Design review of the part shown in the three views and the two pictorial views. Dimensions are in mm from the part's minimum x, y and z. A direction names the side the tool comes from. Give positions to 0.01 mm unless a question says otherwise; leave off trailing zeros. Loops run counter-clockwise (first coordinate to the right, second up) from the corner with the lowest first, then second, coordinate; pieces in that order, holes last. Notation, with made-up numbers: (80.5, -12.75) -> (102.5, -12.75) arc R27 ccw to (102.5, 24.25) -> close; hole circle Ø6 at (-9, -22). An arc over 180 degrees is marked (long way). One line per question, with ' | ' between items. Start each with the question number.
(1) Draft analysis for pull direction Y (two halves, no side actions). For the marked faces 1, 2, 3 and 4, state which applies: +Y half, -Y half, draft (parallel to the pull), parting line (faces both ways), or undercut.
(2) Insertion check: P1, Ø2, axis at y = 11.5, z = 12.5, coming from the -X side; P2, Ø3, axis at x = 59.92, y = 6.35, coming from the +Z side; P3, Ø2, axis at x = 60.5, y = 8, coming from the +Z side; P4, Ø3, axis at y = 8, z = 12.5, coming from the -X side (1 decimal). Each pin has a flat end and moves straight along its axis. Give the tip position at first contact, or say it passes through.
(3) Consider section D-D (y = 9.5). Write out the cut boundary in (x, z).
(4) Consider section C-C (z = 10.25). Write out the cut boundary in (x, y).
(5) Tool access review of the marked faces 5 and 6: name each direction out of +Z, -Z, +X, -X, +Y, -Y from which nothing blocks a thin tool from reaching the whole face with its end or side.
(6) Wall thickness on probe 1 along X at (y, z) = (8.5, 4) (1 decimal); probe 2 along X at (y, z) = (11, 5.75); probe 3 along Z at (x, y) = (61.5, 1.5): over which ranges is each line inside the solid? List them lowest first.
(7) Consider section A-A (y = 6.35). Write out the cut boundary in (x, z).
(8) Consider section B-B (z = 2). Give the number of separate pieces and of enclosed holes in the cut face, and give its area (3 significant figures).
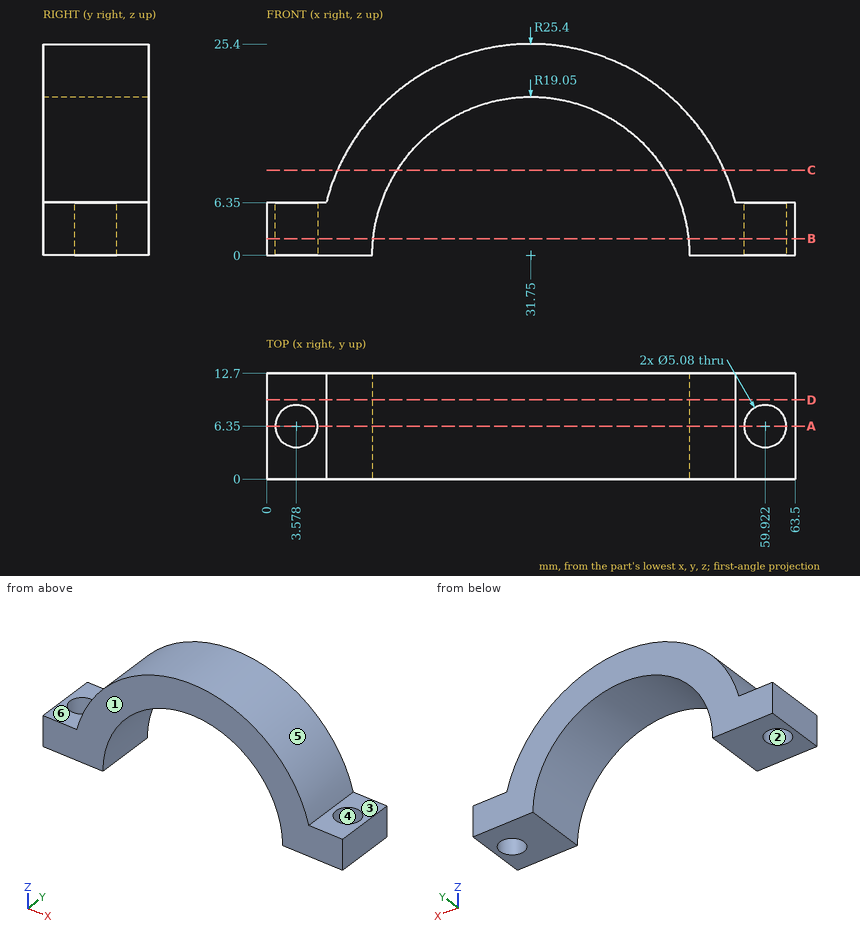
A:
1) face 1: -Y half | face 2: undercut | face 3: draft | face 4: undercut
2) P1: stops at x = 9.1 | P2: passes through | P3: stops at z = 6.35 | P4: stops at x = 8.9
3) outline: (0, 0) -> (12.7, 0) arc R19.05 cw to (50.8, 0) -> (63.5, 0) -> (63.5, 6.35) -> (56.34, 6.35) arc R25.4 ccw to (7.16, 6.35) -> (0, 6.35) -> close
4) outline: (8.51, 0) -> (15.69, 0) -> (15.69, 12.7) -> (8.51, 12.7) -> close; (47.81, 0) -> (54.99, 0) -> (54.99, 12.7) -> (47.81, 12.7) -> close
5) face 5: +Z, +Y, -Y | face 6: +Z, -X, +Y, -Y
6) probe 1: x = 0 to 2.2, 4.9 to 13.1, 50.4 to 58.6, 61.3 to 63.5 | probe 2: x = 0 to 13.59, 49.91 to 63.5 | probe 3: z = 0 to 6.35
7) outline: (0, 0) -> (1.04, 0) -> (1.04, 6.35) -> (0, 6.35) -> close; (6.12, 0) -> (12.7, 0) arc R19.05 cw to (50.8, 0) -> (57.38, 0) -> (57.38, 6.35) -> (56.34, 6.35) arc R25.4 ccw to (7.16, 6.35) -> (6.12, 6.35) -> close; (62.46, 0) -> (63.5, 0) -> (63.5, 6.35) -> (62.46, 6.35) -> close
8) separate pieces: 2 | enclosed holes: 2 | area: 285 mm^2
